Geometry: see drawing. Coordinates: mm, zero at the bounding-box minimum. A direction names the side the tool comes from. Round coordinates to 2 decimals unless told otherwise and drop trailing zeros. Order: outer loops, then holes, each group sorted by start corner. A loop starts at its lowest first (then second) coordinate and runs counter-clockwise, first axis right, second up. Notation, with made-up numbers: (-13.75, 34.5) -> (31.25, 34.5) arc R15 ccw to (31.25, 63.5) -> close; hole circle Ø6 at (74, -39). An arc over 180 degrees is marked (long way). One line per item, written item: value. Start each with the question number.
1) Reachability of the marked faces 1, 2 and 3 from +Z, -Z, +X, -X, +Y, -Y: full face, straight path, thin tool, end or side. Return the list, or none.
2) Section A-A (y = 3.25). Return the cut outline in (x, z).
3) Ray query, L1, parallel to X at y = 6.45, z = 36.5; L2, parallel to X at y = 5.15, z = 3.5; L3, parallel to Z at x = 3, y = 7.25. Return the intervals inside material, ascending.
4) Pin query (flat end, axial travel): P1, Ø2, axis at x = 2.5, z = 3, coming from the -Y side; P2, Ø2, axis at x = 44, z = 35.5, coming from the +Y side; P3, Ø3, axis at y = 10.5, z = 2.5, coming from the -X side; P4, Ø2.5, axis at x = 44.5, z = 36.5, coming from the -Y side. Return the tip coordinate at first contact, or that it passes through.
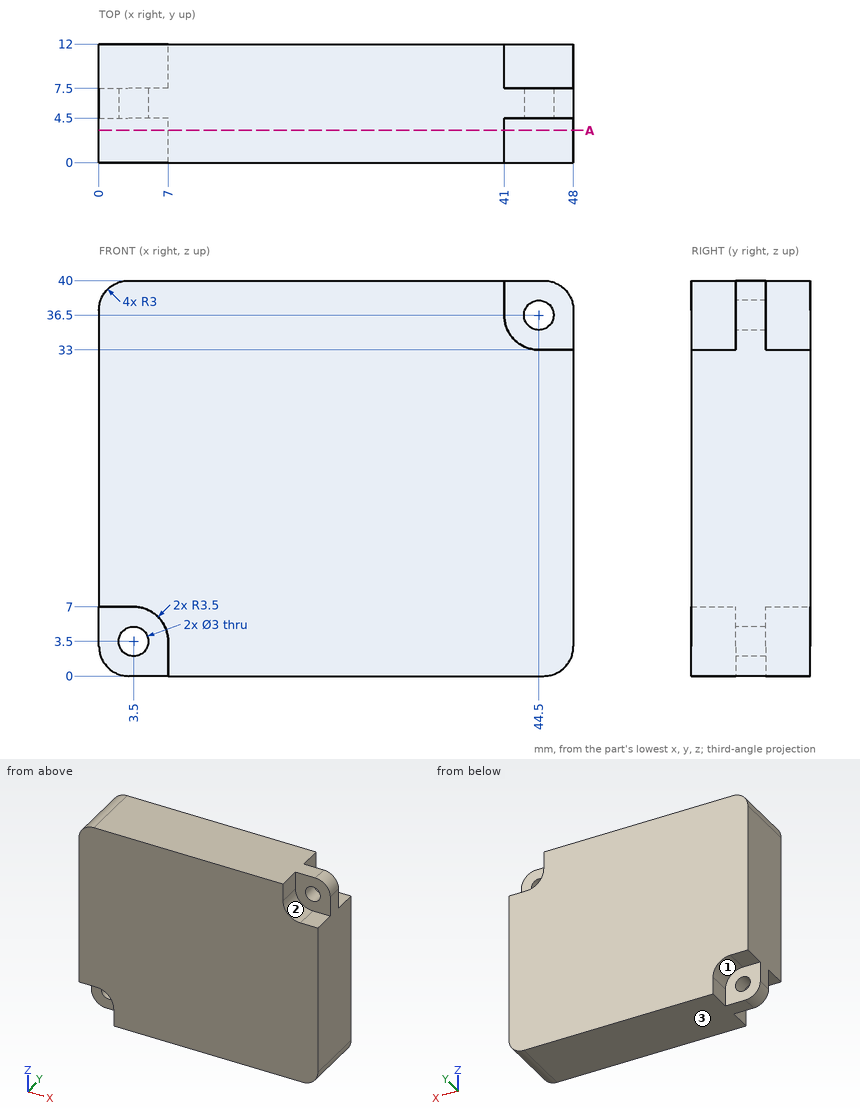
Findings:
1. face 1: -Z, -X, +Y
1. face 2: +Z, +X, -Y
1. face 3: -Z, +X, -X, +Y, -Y
2. outline: (0, 7) -> (3.5, 7) arc R3.5 cw to (7, 3.5) -> (7, 0) -> (45, 0) arc R3 ccw to (48, 3) -> (48, 33) -> (44.5, 33) arc R3.5 cw to (41, 36.5) -> (41, 40) -> (3, 40) arc R3 ccw to (0, 37) -> close
3. L1: 0 to 43, 46 to 48
3. L2: 0 to 2, 5 to 48
3. L3: 0 to 2.09, 4.91 to 40
4. P1: y = 4.5
4. P2: y = 7.5
4. P3: x = 6.96
4. P4: through
